from build123d import *

# Parameters (mm, degrees)
SKETCH2_W           = 50.8
SKETCH2_H           = 160.02
BOSS_EXTRUDE1_DEPTH = 12.7
SKETCH3_R           = 2.4892
CUT_EXTRUDE1_DEPTH  = 169.369624339
FILLET1_R           = 6.35
SKETCH4_W           = 3.175
SKETCH4_H           = 33.02
CUT_EXTRUDE2_DEPTH  = 169.369624339
FILLET3_R           = 6.35


with BuildPart() as part:
    # Sketch2 → Boss-Extrude1 (new body)
    with BuildSketch(Plane.XY):
        with Locations((25.4, 80.01)):
            Rectangle(SKETCH2_W, SKETCH2_H)
    extrude(amount=-BOSS_EXTRUDE1_DEPTH)

    # Sketch3 → Cut-Extrude1 (cut, through all)
    with BuildSketch(Plane.XY):
        with Locations((12.7, 147.32)):
            Circle(SKETCH3_R)
        with Locations((38.1, 147.32)):
            Circle(SKETCH3_R)
        with Locations((12.7, 114.3)):
            Circle(SKETCH3_R)
        with Locations((12.7, 101.6)):
            Circle(SKETCH3_R)
        with Locations((12.7, 88.9)):
            Circle(SKETCH3_R)
        with Locations((12.7, 76.2)):
            Circle(SKETCH3_R)
        with Locations((12.7, 63.5)):
            Circle(SKETCH3_R)
        with Locations((38.1, 101.6)):
            Circle(SKETCH3_R)
        with Locations((38.1, 88.9)):
            Circle(SKETCH3_R)
        with Locations((38.1, 76.2)):
            Circle(SKETCH3_R)
        with Locations((38.1, 63.5)):
            Circle(SKETCH3_R)
        with Locations((38.1, 114.3)):
            Circle(SKETCH3_R)
        with Locations((12.7, 50.8)):
            Circle(SKETCH3_R)
        with Locations((12.7, 38.1)):
            Circle(SKETCH3_R)
        with Locations((12.7, 25.4)):
            Circle(SKETCH3_R)
        with Locations((12.7, 12.7)):
            Circle(SKETCH3_R)
        with Locations((38.1, 50.8)):
            Circle(SKETCH3_R)
        with Locations((38.1, 38.1)):
            Circle(SKETCH3_R)
        with Locations((38.1, 25.4)):
            Circle(SKETCH3_R)
        with Locations((38.1, 12.7)):
            Circle(SKETCH3_R)
    extrude(amount=-CUT_EXTRUDE1_DEPTH, mode=Mode.SUBTRACT)

    # Fillet1
    fillet1_edges = [part.edges().sort_by_distance(p)[0] for p in [
        (0, 160.02, -6.35),
        (50.8, 160.02, -6.35),
        (50.8, 0, -6.35),
        (0, 0, -6.35),
    ]]
    fillet(fillet1_edges, radius=FILLET1_R)

    # Sketch4 → Cut-Extrude2 (cut, through all)
    with BuildSketch(Plane.ZY):
        with Locations((-1.5875, 143.51)):
            Rectangle(SKETCH4_W, SKETCH4_H)
    extrude(amount=-CUT_EXTRUDE2_DEPTH, mode=Mode.SUBTRACT)

    # Fillet3
    fillet3_edges = [part.edges().sort_by_distance(p)[0] for p in [
        (0, 127, -1.5875),
        (50.8, 127, -1.5875),
    ]]
    fillet(fillet3_edges, radius=FILLET3_R)


solid = part.part
Geometry check sheet. Reference: the model listing, model coordinates, mm. A direction names the side the tool comes from. Coordinates: 2 decimals unless noted, no trailing zeros. Order: outer loops, then holes, each group sorted by start corner. A loop starts at its lowest first (then second) coordinate and runs counter-clockwise, first axis right, second up. Notation, with made-up numbers: (-21, 36) -> (-9, 36) arc R34 ccw to (-9, 69) -> close; hole circle Ø1 at (69.5, 46.25). An arc over 180 degrees is marked (long way). Use a Markdown table: item, result. Add a question column.
1. Go/stop test with a flat-tipped pin: pin 1 Ø12 at (x, y) = (28, 139.5) entering from +Z (3 decimals). Record where the tip stops, or that it passes through.
2. Cross-section at C-C (x = 20). Enter the section's corners in (y, z) (3 decimals).
3. Material ranges on L1, parallel to X at y = 51, z = -4.75; L2, parallel to X at y = 65, z = -2; L3, parallel to Y at x = 21, z = -2.75, recorded low to high.
4. Cross-section at D-D (y = 50.8). Enter the section's corners in (x, z), and give its area (3 significant figures).
5. Mould release check, pull along X, two halves, no side actions. Record for faces 3 (the face through (12.38, 27.87, -6.26)), 4 (the face through (25, 127, -2)), 5 (the face through (1.81, 1.91, -6.44)): pulls with the +X half, pulls with the -X half, needs draft (parallel to the pull), parting line crosses it, or undercut.
6. Cross-section at A-A (z = -8). Give the number of separate pieces and of enclosed holes in the cut face, and give its area (3 significant figures).
7. Cross-section at B-B (y = 147.32). Enter the section's corners in (x, z) (3 decimals), and give its area (3 significant figures).
8. Set-up check for faces 1 (the face through (36.12, 36.59, -6.26)), 2 (the face through (48.89, 125.19, -1.61)): record each of +Z, -Z, +X, -X, +Y, -Y from which the full face is reachable in a straight line by a thin tool's end or side.
Filled sheet:
| question | item | result |
|---|---|---|
| 1 | pin 1 | z = -3.175 |
| 2 | outline | (0, -12.7) -> (160.02, -12.7) -> (160.02, -3.175) -> (127, -3.175) -> (127, 0) -> (0, 0) -> close |
| 3 | L1 | 0 to 10.22, 15.18 to 35.62, 40.58 to 50.8 |
| 3 | L2 | 0 to 10.71, 14.69 to 36.11, 40.09 to 50.8 |
| 3 | L3 | 0 to 127 |
| 4 | outline | (0, -12.7) -> (10.21, -12.7) -> (10.21, 0) -> (0, 0) -> close; (15.19, -12.7) -> (35.61, -12.7) -> (35.61, 0) -> (15.19, 0) -> close; (40.59, -12.7) -> (50.8, -12.7) -> (50.8, 0) -> (40.59, 0) -> close |
| 4 | area | 519 mm2 |
| 5 | face 3 | undercut |
| 5 | face 4 | needs draft |
| 5 | face 5 | pulls with the -X half |
| 6 | separate pieces | 1 |
| 6 | enclosed holes | 20 |
| 6 | area | 7,710 mm2 |
| 7 | outline | (0, -12.7) -> (10.211, -12.7) -> (10.211, -3.175) -> (0, -3.175) -> close; (15.189, -12.7) -> (35.611, -12.7) -> (35.611, -3.175) -> (15.189, -3.175) -> close; (40.589, -12.7) -> (50.8, -12.7) -> (50.8, -3.175) -> (40.589, -3.175) -> close |
| 7 | area | 389 mm2 |
| 8 | face 1 | +Z, -Z |
| 8 | face 2 | +Z, +X, +Y |
